For this review, take the finished solid that the model builds, in its own axes (mm). Face numbers are marked on the shaded views. A direction names the side the tool comes from. Coordinates: 2 decimals unless noted, no trailing zeros. Loops run counter-clockwise (first coordinate to the right, second up) from the corner with the lowest first, then second, coordinate; pieces in that order, holes last.
1. Take a section at C-C, the plane x = -1.5. State the section outline as (y, z) points, then the cut area to 3 significant figures.
2. Clearance check with flat-ended pins moving along their axes: P1, Ø3, axis at x = -27.9, y = -24.75, coming from the -Z side; P2, Ø0.7, axis at x = 31.5, y = 17.5, coming from the +Z side; P3, Ø2.5, axis at x = -6.5, z = 5, coming from the -Y side; P4, Ø2.5, axis at x = -9, z = 3.5, coming from the +Y side. State where each tip first meets the part, or that it passes through.
3. Take a section at B-B, the plane y = -2. State the section outline as (x, z) points.
4. Mouldability with a two-part tool opening along Y and no side actions: class the marked faces 1, 2 and 3 as pulls with the +Y half, pulls with the -Y half, needs draft (parallel to the pull), parting line crosses it, or undercut.
5. To check wall thickness, follow probe 1 along Y at (x, z) = (-15.5, 5.25); probe 2 along X at (y, z) = (9, 2.75); probe 3 along Y at (x, z) = (24.5, 1.5). State the ranges of each line that lie inside material, in increasing order.
6. Take a section at A-A, the plane x = -27.9. State the section outline as (y, z) points, then the cut area to 3 significant figures.
7. Machinability: for the marked faces 4, 5 and 6, which of the approach directions +Z, -Z, +X, -X, +Y, -Y give a long, thin tool a straight path to every point of the face, cutting with its end or side? Answer none if there is none.
8. Take a section at D-D, the plane z = 7. State the section outline as (x, y) points (3 decimals).
```python
from build123d import *

# Parameters (mm, degrees)
SKETCH_R     = 1.7
SKETCH_W     = 61.2
SKETCH_H     = 38
PAD_DEPTH    = 8
SKETCH001_W  = 2
SKETCH001_H  = 4.5
POCKET_DEPTH = 1.3


with BuildPart() as part:
    # Sketch → Pad (new body)
    with BuildSketch(Plane.XY):
        with BuildLine():
            Line((-31.9, 20.3), (-31.9, -20.3))
            Line((-31.9, -20.3), (-30.835954, -25.366584))
            ThreePointArc((-30.835954, -25.366584), (-27.229087, -27.674017), (-24.988925, -24.024987))
            ThreePointArc((-22.077844, -20.3), (-24.441629, -21.4527), (-24.988925, -24.024987))
            Line((22.077844, -20.3), (-22.077844, -20.3))
            ThreePointArc((24.988925, -24.024987), (24.441629, -21.452699), (22.077844, -20.3))
            ThreePointArc((24.988925, -24.024987), (27.229087, -27.674017), (30.835954, -25.366583))
            Line((31.9, -20.3), (30.835954, -25.366583))
            Line((31.9, 20.3), (31.9, -20.3))
            Line((31.9, 20.3), (30.835954, 25.366583))
            ThreePointArc((30.835954, 25.366583), (27.229093, 27.674018), (24.988922, 24.025))
            ThreePointArc((22.077844, 20.3), (24.441633, 21.452705), (24.988922, 24.025))
            Line((-22.077844, 20.3), (22.077844, 20.3))
            ThreePointArc((-24.988922, 24.025), (-24.441633, 21.452705), (-22.077844, 20.3))
            ThreePointArc((-24.988922, 24.025), (-27.229093, 27.674018), (-30.835954, 25.366584))
            Line((-31.9, 20.3), (-30.835954, 25.366584))
        make_face()
        with Locations((-27.9, -24.75)):
            Circle(SKETCH_R, mode=Mode.SUBTRACT)
        with Locations((27.9, -24.75)):
            Circle(SKETCH_R, mode=Mode.SUBTRACT)
        with Locations((27.9, 24.75)):
            Circle(SKETCH_R, mode=Mode.SUBTRACT)
        with Locations((-27.9, 24.75)):
            Circle(SKETCH_R, mode=Mode.SUBTRACT)
        Rectangle(SKETCH_W, SKETCH_H, mode=Mode.SUBTRACT)
    extrude(amount=PAD_DEPTH)

    # Sketch001 → Pocket (cut)
    with BuildSketch(Plane.YZ.offset(31.9)):
        with Locations((18, 5.75)):
            Rectangle(SKETCH001_W, SKETCH001_H)
    extrude(amount=-POCKET_DEPTH, mode=Mode.SUBTRACT)


solid = part.part
```
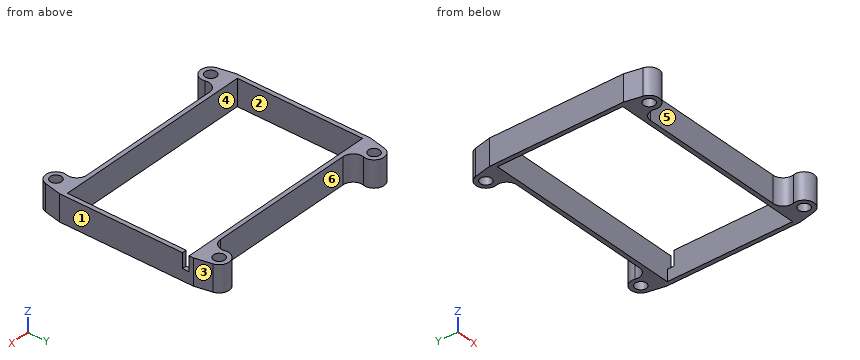
Results list:
1. outline: (-20.3, 0) - (-19, 0) - (-19, 8) - (-20.3, 8) - close; (19, 0) - (20.3, 0) - (20.3, 8) - (19, 8) - close
1. area: 20.8 mm2
2. P1: passes through
2. P2: stops at z = 3.5
2. P3: stops at y = -20.3
2. P4: stops at y = 20.3
3. outline: (-31.9, 0) - (-30.6, 0) - (-30.6, 8) - (-31.9, 8) - close; (30.6, 0) - (31.9, 0) - (31.9, 8) - (30.6, 8) - close
4. face 1: needs draft
4. face 2: undercut
4. face 3: pulls with the +Y half
5. probe 1: y = -20.3 to -19, 19 to 20.3
5. probe 2: x = -31.9 to -30.6, 30.6 to 31.9
5. probe 3: y = -21.53 to -19, 19 to 21.53
6. outline: (-27.75, 0) - (-26.45, 0) - (-26.45, 8) - (-27.75, 8) - close; (-23.05, 0) - (-19, 0) - (-19, 8) - (-23.05, 8) - close; (19, 0) - (23.05, 0) - (23.05, 8) - (19, 8) - close; (26.45, 0) - (27.75, 0) - (27.75, 8) - (26.45, 8) - close
6. area: 85.6 mm2
7. face 4: +Z, -Z
7. face 5: +Z, -Z, -Y
7. face 6: +Z, -Z, +Y
8. outline: (-31.9, -20.3) - (-30.836, -25.367) arc R3 ccw (long way) to (-24.989, -24.025) arc R3 cw to (-22.078, -20.3) - (22.078, -20.3) arc R3 cw to (24.989, -24.025) arc R3 ccw (long way) to (30.836, -25.367) - (31.9, -20.3) - (31.9, 17) - (30.6, 17) - (30.6, -19) - (-30.6, -19) - (-30.6, 19) - (31.9, 19) - (31.9, 20.3) - (30.836, 25.367) arc R3 ccw (long way) to (24.989, 24.025) arc R3 cw to (22.078, 20.3) - (-22.078, 20.3) arc R3 cw to (-24.989, 24.025) arc R3 ccw (long way) to (-30.836, 25.367) - (-31.9, 20.3) - close; hole circle Ø3.4 at (-27.9, -24.75); hole circle Ø3.4 at (-27.9, 24.75); hole circle Ø3.4 at (27.9, -24.75); hole circle Ø3.4 at (27.9, 24.75)
